Geometry check sheet. Reference: the model listing, model coordinates, mm. Face numbers are marked on the shaded views. Coordinates: 2 decimals unless noted, no trailing zeros. Loops run counter-clockwise (first coordinate to the right, second up) from the corner with the lowest first, then second, coordinate; pieces in that order, holes last. Notation, with made-up numbers: M 73.25,88 L 113.25,88 A23 ccw 113.25,120 Z; hole C 17,27 d4. An arc over 180 degrees is marked long. Use CSV: the item, a comma, the result in double quotes.
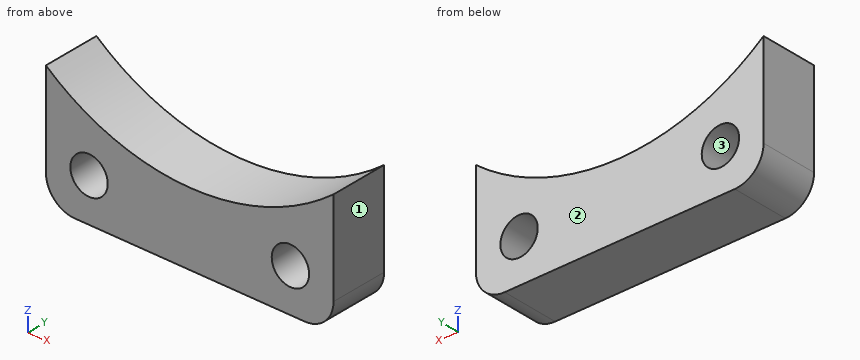
```python
from build123d import *

# Parameters (mm, degrees)
BOSS_EXTRU_1_DEPTH      = 10
CONG_1_R                = 5
ESQUISSE3_R             = 3.25
ENL_V_MAT_EXTRU_1_DEPTH = 11


with BuildPart() as part:
    # Esquisse1 → Boss.-Extru.1 (new body)
    with BuildSketch(Plane(origin=(0, 0, 0), x_dir=(1, 0, 0), z_dir=(0, 1, 0))):
        with BuildLine():
            Line((25, 31.224989992), (25, 52.5))
            Line((25, 52.5), (-25, 52.5))
            Line((-25, 52.5), (-25, 31.224989992))
            ThreePointArc((-25, 31.224989992), (0, 40), (25, 31.224989992))
        make_face()
    extrude(amount=BOSS_EXTRU_1_DEPTH)

    # Congé1
    cong_1_edges = [part.edges().sort_by_distance(p)[0] for p in [
        (-25, 5, -52.5),
        (25, 5, -52.5),
    ]]
    fillet(cong_1_edges, radius=CONG_1_R)

    # Esquisse3 → Enlèv. mat.-Extru.1 (cut, through all)
    with BuildSketch(Plane(origin=(0, 10, 0), x_dir=(1, 0, 0), z_dir=(0, 1, 0))):
        with Locations(Location((-17.5, 45, 0), (0, 0, 270))):  # turned: the seam where the file's is
            Circle(ESQUISSE3_R)
        with Locations(Location((17.5, 45, 0), (0, 0, 270))):  # turned: the seam where the file's is
            Circle(ESQUISSE3_R)
    extrude(amount=-ENL_V_MAT_EXTRU_1_DEPTH, mode=Mode.SUBTRACT)


solid = part.part
```
1. Section check C-C, the plane x = -19. Record the cut outline in (y, z), plus the area to 3 significant figures.
The answers:
outline,"M 0,-52.5 L 10,-52.5 L 10,-47.88 L 0,-47.88 Z; M 0,-42.12 L 10,-42.12 L 10,-35.2 L 0,-35.2 Z"
area,"115 mm^2"
2. Section check B-B, the plane y = 5.5. Record the cut outline in (x, z).
The answers:
outline,"M -25,-47.5 A5 ccw -20,-52.5 L 20,-52.5 A5 ccw 25,-47.5 L 25,-31.22 A40 cw -25,-31.22 Z; hole C -17.5,-45 d6.5; hole C 17.5,-45 d6.5"
3. Section check D-D, the plane z = -34. Record the cut outline in (x, y), plus the area to 3 significant figures.
The answers:
outline,"M -25,0 L -21.07,0 L -21.07,10 L -25,10 Z; M 21.07,0 L 25,0 L 25,10 L 21.07,10 Z"
area,"78.6 mm^2"
4. Section check A-A, the plane z = -45. Record the cut outline in (x, y).
The answers:
outline,"M -25,0 L -20.75,0 L -20.75,10 L -25,10 Z; M -14.25,0 L 14.25,0 L 14.25,10 L -14.25,10 Z; M 20.75,0 L 25,0 L 25,10 L 20.75,10 Z"
5. Thickness scan on line 1 (X direction, y = 4.75, z = -45); line 2 (X direction, y = 2.5, z = -44); line 3 (X direction, y = 1.25, z = -33). Record the ranges inside material, lowest first. Write a range as [from, to].
The answers:
line 1,"[-25, -20.75], [-14.25, 14.25], [20.75, 25]"
line 2,"[-25, -20.59], [-14.41, 14.41], [20.59, 25]"
line 3,"[-25, -22.61], [22.61, 25]"
6. Release check for a two-part mould opening along X. For the marked faces 1, 2 and 3 record: +X half, -X half, draft (parallel to the pull), parting line (faces both ways), or undercut.
The answers:
face 1,"+X half"
face 2,"draft"
face 3,"undercut"
